Can you work these out from the drawing? Everything is in mm from the part's minimum corner. A direction names the side the tool comes from. Give positions to 0.01 mm unless a question says otherwise; leave off trailing zeros. Loops run counter-clockwise (first coordinate to the right, second up) from the corner with the lowest first, then second, coordinate; pieces in that order, holes last.
Q1. If we section it at D-D (x = 11.5): Please give me the cut outline in (y, z) (1 decimal).
Q2. Will this pin go through, and if not, where does the flat tip stop? P1, Ø1.2, axis at x = 11, z = 5.5, coming from the -Y side.
Q3. I need wall thicknesses on line 1 (X direction, y = 4.25, z = 2.94); line 2 (Z direction, x = 21.94, y = 3.25); line 3 (X direction, y = 3, z = 3.25). Which ranges of each line are inside material? Lowest first, please.
Q4. If we section it at C-C (y = 5.5): Please give me the cut outline in (x, z), plus the area to 3 significant figures.
Q5. If we section it at B-B (y = 1.5): Please give me the cut outline in (x, z).
Q6. We'd pull the mould along X, two halves only. Please class the marked faces 1, 2 and 3: +X half, -X half, draft (parallel to the pull), parting line (faces both ways), or undercut.
Q7. If we section it at A-A (x = 3.06): Please give me the cut outline in (y, z).
Q8. For the marked faces 4, 5 and 6, which set-ups out of +Z, -Z, +X, -X, +Y, -Y let a thin tool reach every point of the face, with its end or its side?
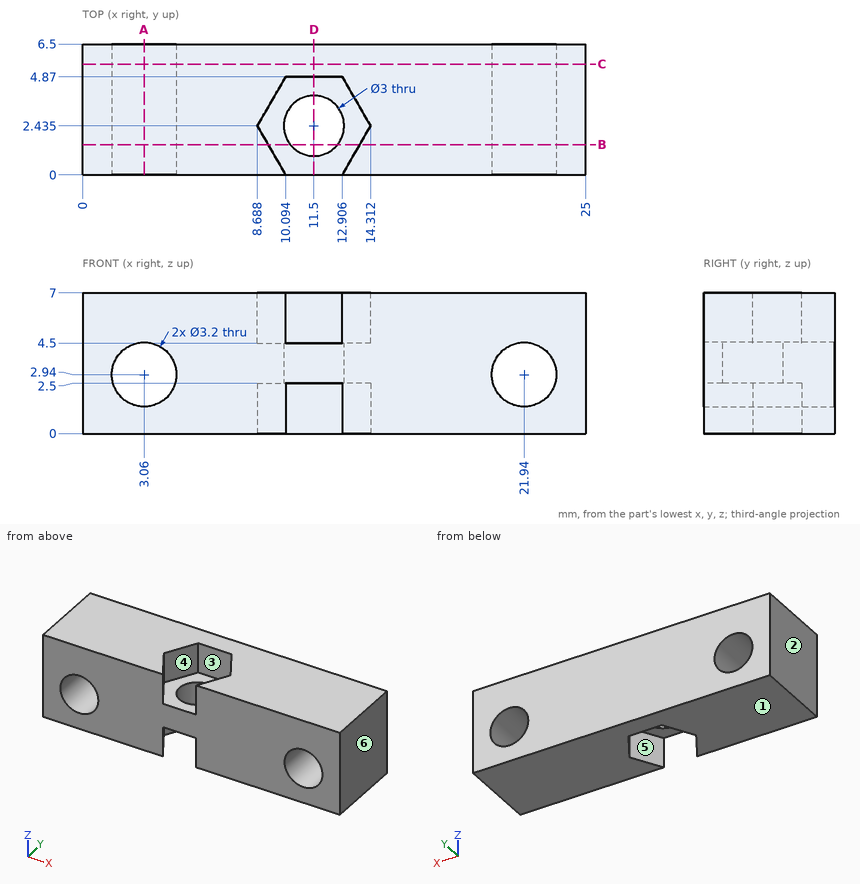
Check sheet entries:
1. outline: (0, 2.5) - (0.9, 2.5) - (0.9, 4.5) - (0, 4.5) - close; (3.9, 2.5) - (4.9, 2.5) - (4.9, 0) - (6.5, 0) - (6.5, 7) - (4.9, 7) - (4.9, 4.5) - (3.9, 4.5) - close
2. P1: stops at y = 4.87
3. line 1: x = 0 to 1.46, 4.66 to 20.34, 23.54 to 25
3. line 2: z = 0 to 1.34, 4.54 to 7
3. line 3: x = 0 to 1.49, 4.63 to 10.11, 12.89 to 20.37, 23.51 to 25
4. outline: (0, 0) - (25, 0) - (25, 7) - (0, 7) - close; hole circle Ø3.2 at (3.06, 2.94); hole circle Ø3.2 at (21.94, 2.94)
4. area: 159 mm2
5. outline: (0, 0) - (9.23, 0) - (9.23, 2.5) - (10.33, 2.5) - (10.33, 4.5) - (9.23, 4.5) - (9.23, 7) - (0, 7) - close; (12.67, 2.5) - (13.77, 2.5) - (13.77, 0) - (25, 0) - (25, 7) - (13.77, 7) - (13.77, 4.5) - (12.67, 4.5) - close; hole circle Ø3.2 at (3.06, 2.94); hole circle Ø3.2 at (21.94, 2.94)
6. face 1: draft
6. face 2: -X half
6. face 3: undercut
7. outline: (0, 0) - (6.5, 0) - (6.5, 1.34) - (0, 1.34) - close; (0, 4.54) - (6.5, 4.54) - (6.5, 7) - (0, 7) - close
8. face 4: +Z
8. face 5: -Z
8. face 6: +Z, -Z, +X, +Y, -Y
